from build123d import *

# Parameters (mm, degrees)
F0_W     = 25.4
F0_H     = 25.4
F1_DEPTH = 25.4
F2_R     = 9.525
F3_DEPTH = 22.86
F4_R     = 7.116494
F5_DEPTH = 2.541
F6_R     = 1.27
F7_DEPTH = 25.401


with BuildPart() as f1:
    # F0 (on Top) → F1 (new body)
    with BuildSketch(Plane.XY):
        with Locations((12.7, 12.7)):
            Rectangle(F0_W, F0_H)
    extrude(amount=F1_DEPTH)

    # F2 (on face) → F3 (cut)
    with BuildSketch(Plane.XY.offset(25.4)):
        with Locations((12.7, 12.7)):
            Circle(F2_R)
    extrude(amount=-F3_DEPTH, mode=Mode.SUBTRACT)

    # F4 (on face) → F5 (cut, through all)
    with BuildSketch(Plane.XY.offset(2.54)):
        with Locations((12.7, 12.7)):
            Circle(F4_R)
    extrude(amount=-F5_DEPTH, mode=Mode.SUBTRACT)

    # F6 (on face) → F7 (cut, through all)
    with BuildSketch(Plane.XY.offset(25.4)):
        with Locations((21.844, 3.556)):
            Circle(F6_R)
        with Locations((21.844, 21.844)):
            Circle(F6_R)
        with Locations((3.556, 21.844)):
            Circle(F6_R)
        with Locations((3.556, 3.556)):
            Circle(F6_R)
    extrude(amount=-F7_DEPTH, mode=Mode.SUBTRACT)


solid = f1.part
Can you work these out from the model? Positions are in its coordinate system, mm. A direction names the side the tool comes from. Give positions to 0.01 mm unless a question says otherwise; leave off trailing zeros. Order: outer loops, then holes, each group sorted by start corner. A loop starts at its lowest first (then second) coordinate and runs counter-clockwise, first axis right, second up. Notation, with made-up numbers: M 47.25,-40 L 88.25,-40 A20 ccw 88.25,-27 Z; hole C -12,30 d11. An arc over 180 degrees is marked long. Use a Markdown table: item, result. Add a question column.
Item 1: Suppose I cut it at C-C (x = 21). List the corners of the cut face in (y, z) for me.
Item 2: We'd pull the mould along Y, two halves only. Please class faces 3 (the flat face through (13, 0, 13)), 4 (the flat face through (18, 4, 25.4)), 5 (the cylindrical face through (3.391, 4.815, 12.878)): +Y half, -Y half, draft (parallel to the pull), parting line (faces both ways), or undercut.
Item 3: For faces 1 (the cylindrical face through (3.3, 20.6, 12.9)), 2 (the cylindrical face through (10.64, 3.4, 14.13)), which set-ups out of +Z, -Z, +X, -X, +Y, -Y let a thin tool reach every point of the face, with its end or its side?
Item 4: If I drill on L1, parallel to Y at x = 2.5, z = 6.5; L2, parallel to Y at x = 4, z = 9, over which ranges is the centre line in solid material (lowest first)? Write a range as [from, to].
Item 5: Suppose I cut it at A-A (y = 12.7). List the corners of the cut face in (x, z) for me (1 decimal), then the cut area to 3 significant figures.
Item 6: Suppose I cut it at B-B (x = 17.5). List the corners of the cut face in (y, z) for me.
Item 7: Will these pins go through, and if not, where does the flat tip stop? pin 1 (1.5 mm diameter, centred on x = 3.556, y = 21.844, fed in from +Z); pin 2 (15 mm diameter, centred on x = 13.5, y = 9, fed in from +Z).
Item 8: Suppose I cut it at D-D (z = 22.25). List the corners of the cut face in (x, y) for me (3 decimals).
Answer sheet:
| question | item | result |
|---|---|---|
| 1 | outline | M 0,0 L 2.61,0 L 2.61,25.4 L 0,25.4 Z; M 4.5,0 L 20.9,0 L 20.9,25.4 L 17.37,25.4 L 17.37,2.54 L 8.03,2.54 L 8.03,25.4 L 4.5,25.4 Z; M 22.79,0 L 25.4,0 L 25.4,25.4 L 22.79,25.4 Z |
| 2 | face 3 | -Y half |
| 2 | face 4 | draft |
| 2 | face 5 | undercut |
| 3 | face 1 | +Z, -Z |
| 3 | face 2 | +Z |
| 4 | L1 | y = [0, 2.85], [4.26, 21.14], [22.55, 25.4] |
| 4 | L2 | y = [0, 2.37], [4.75, 8.82], [16.58, 20.65], [23.03, 25.4] |
| 5 | outline | M 0,0 L 5.6,0 L 5.6,2.5 L 3.2,2.5 L 3.2,25.4 L 0,25.4 Z; M 19.8,0 L 25.4,0 L 25.4,25.4 L 22.2,25.4 L 22.2,2.5 L 19.8,2.5 Z |
| 5 | area | 174 mm² |
| 6 | outline | M 0,0 L 7.45,0 L 7.45,2.54 L 4.47,2.54 L 4.47,25.4 L 0,25.4 Z; M 17.95,0 L 25.4,0 L 25.4,25.4 L 20.93,25.4 L 20.93,2.54 L 17.95,2.54 Z |
| 7 | pin 1 | passes through |
| 7 | pin 2 | stops at z = 25.4 |
| 8 | outline | M 0,0 L 25.4,0 L 25.4,25.4 L 0,25.4 Z; hole C 3.556,3.556 d2.54; hole C 3.556,21.844 d2.54; hole C 12.7,12.7 d19.05; hole C 21.844,3.556 d2.54; hole C 21.844,21.844 d2.54 |
